Verification items for the finished model (mm, model axes). Face numbers are marked on the shaded views. A direction names the side the tool comes from. Round coordinates to 2 decimals unless told otherwise and drop trailing zeros. Write each loop counter-clockwise with the first axis right and the second up, starting at its lowest first coordinate (ties: lowest second). Pieces come first, ordered by that corner, then holes. Notation, with made-up numbers: (-11, 83) - (40, 83) arc R21 cw to (40, 88) - close; hole circle Ø1 at (57, 29.25). An arc over 180 degrees is marked (long way). Answer as a JSON object with one key per item and string values.
```python
from build123d import *

# Parameters (mm, degrees)
BOSS_EXTRUDE1_DEPTH = 5
SKETCH6_R           = 7
SKETCH6_R_2         = 2.25
CUT_EXTRUDE1_DEPTH  = 91.496055715
BOSS_EXTRUDE2_DEPTH = 10
SKETCH11_R          = 2.59
CUT_EXTRUDE3_DEPTH  = 3
SKETCH16_R          = 1.5
CUT_EXTRUDE6_DEPTH  = 119.415100811
SKETCH24_W          = 10
SKETCH24_H          = 50
BOSS_EXTRUDE8_DEPTH = 40
SKETCH25_R          = 7
CUT_EXTRUDE10_DEPTH = 132.23313644
SKETCH26_R          = 1.55
CUT_EXTRUDE11_DEPTH = 132.23313644


with BuildPart() as part:
    # Sketch3 → Boss-Extrude1 (new, symmetric)
    with BuildSketch(Plane.XY):
        with BuildLine():
            Line((0, 20), (87.69, 20))
            Line((87.69, 20), (87.69, -20))
            Line((87.69, -20), (0, -20))
            ThreePointArc((0, -20), (-20, 0), (0, 20))
        make_face()
    extrude(amount=BOSS_EXTRUDE1_DEPTH, both=True)

    # Sketch6 → Cut-Extrude1 (cut, through all)
    with BuildSketch(Plane.XY.offset(5)):
        with Locations((20, 0)):
            Circle(SKETCH6_R)
        with Locations((20, 11)):
            Circle(SKETCH6_R_2)
        with Locations((31, 0)):
            Circle(SKETCH6_R_2)
        with Locations((20, -11)):
            Circle(SKETCH6_R_2)
        with Locations((9, 0)):
            Circle(SKETCH6_R_2)
    extrude(amount=-CUT_EXTRUDE1_DEPTH, mode=Mode.SUBTRACT)

    # Sketch9 → Boss-Extrude2 (add)
    with BuildSketch(Plane(origin=(87.69, 0, 0), x_dir=(0, 0, -1), z_dir=(1, 0, 0))):
        Polygon((5, 20), (45, 20), (45, -20), (5, -20), (-5, -20), (-5, 20), align=None)
    extrude(amount=-BOSS_EXTRUDE2_DEPTH)

    # Sketch11 → Cut-Extrude3 (cut)
    with BuildSketch(Plane.XY.offset(5)):
        with Locations((-12, -1.375)):
            Circle(SKETCH11_R)
    extrude(amount=-CUT_EXTRUDE3_DEPTH, mode=Mode.SUBTRACT)

    # Sketch16 → Cut-Extrude6 (cut, through all)
    with BuildSketch(Plane(origin=(87.69, 0, 0), x_dir=(0, 0, -1), z_dir=(1, 0, 0))):
        with Locations((20, 16)):
            Circle(SKETCH16_R)
        with Locations((20, -2)):
            Circle(SKETCH16_R)
    extrude(amount=-CUT_EXTRUDE6_DEPTH, mode=Mode.SUBTRACT)

    # Sketch24 → Boss-Extrude8 (add)
    with BuildSketch(Plane(origin=(0, -20, 0), x_dir=(-1, 0, 0), z_dir=(0, -1, 0))):
        with Locations((-82.69, 20)):
            Rectangle(SKETCH24_W, SKETCH24_H)
    extrude(amount=BOSS_EXTRUDE8_DEPTH)

    # Sketch25 → Cut-Extrude10 (cut, through all)
    with BuildSketch(Plane(origin=(87.69, 0, 0), x_dir=(0, 0, -1), z_dir=(1, 0, 0))):
        with Locations((20, -40)):
            Circle(SKETCH25_R)
    extrude(amount=-CUT_EXTRUDE10_DEPTH, mode=Mode.SUBTRACT)

    # Sketch26 → Cut-Extrude11 (cut, through all)
    with BuildSketch(Plane(origin=(87.69, 0, 0), x_dir=(0, 0, -1), z_dir=(1, 0, 0))):
        with Locations((2.78, -24.223522787)):
            Circle(SKETCH26_R)
        with Locations((37.22, -24.223522787)):
            Circle(SKETCH26_R)
        with Locations((37.22, -55.223522787)):
            Circle(SKETCH26_R)
        with Locations((2.78, -55.223522787)):
            Circle(SKETCH26_R)
    extrude(amount=-CUT_EXTRUDE11_DEPTH, mode=Mode.SUBTRACT)


solid = part.part
```
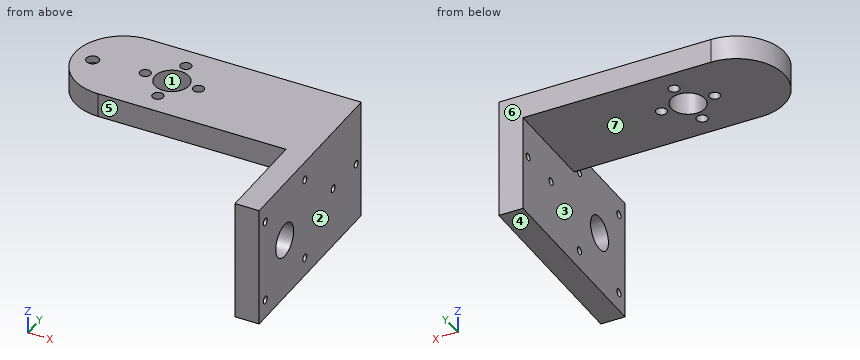
1. Cross-section at D-D (y = 16). Record the boundary of the cut face in (x, z), plus the area to 3 significant figures.
Completed:
{"outline": "(-12, -5) - (77.69, -5) - (77.69, -18.5) - (87.69, -18.5) - (87.69, 5) - (-12, 5) - close; (77.69, -45) - (87.69, -45) - (87.69, -21.5) - (77.69, -21.5) - close", "area": "1,370 mm^2"}
2. Material ranges on probe 1 along Y at (x, z) = (20, 1.5); probe 2 along Y at (x, z) = (80.5, -2.78); probe 3 along Z at (x, y) = (77, -17), recorded low to high. Write a range as from..to.
Completed:
{"probe 1": "y = -20..-13.25, -8.75..-7, 7..8.75, 13.25..20", "probe 2": "y = -60..-56.77, -53.67..-25.77, -22.67..20", "probe 3": "z = -5..5"}
3. Cross-section at B-B (x = 31). Record the boundary of the cut face in (y, z).
Completed:
{"outline": "(-20, -5) - (-2.25, -5) - (-2.25, 5) - (-20, 5) - close; (2.25, -5) - (20, -5) - (20, 5) - (2.25, 5) - close"}
4. Cross-section at A-A (z = -2.78). Record the boundary of the cut face in (x, y).
Completed:
{"outline": "(0, -20) - (77.69, -20) - (77.69, -22.67) - (87.69, -22.67) - (87.69, 20) - (0, 20) arc R20 ccw to start; (77.69, -60) - (87.69, -60) - (87.69, -56.77) - (77.69, -56.77) - close; (77.69, -53.67) - (87.69, -53.67) - (87.69, -25.77) - (77.69, -25.77) - close; hole circle Ø4.5 at (9, 0); hole circle Ø14 at (20, 0); hole circle Ø4.5 at (20, -11); hole circle Ø4.5 at (20, 11); hole circle Ø4.5 at (31, 0)"}
5. Cross-section at C-C (z = -20). Record the boundary of the cut face in (x, y), plus the area to 3 significant figures.
Completed:
{"outline": "(77.69, -60) - (87.69, -60) - (87.69, -47) - (77.69, -47) - close; (77.69, -33) - (87.69, -33) - (87.69, -3.5) - (77.69, -3.5) - close; (77.69, -0.5) - (87.69, -0.5) - (87.69, 14.5) - (77.69, 14.5) - close; (77.69, 17.5) - (87.69, 17.5) - (87.69, 20) - (77.69, 20) - close", "area": "600 mm^2"}
6. Access from +Z, -Z, +X, -X, +Y, -Y to the whole of each face (thin tool, end or side, straight path). Record for the marked faces 5, 6 and 7.
Completed:
{"face 5": "+Z, -Z, -X, -Y", "face 6": "+Z, -Z, +X, -X, +Y", "face 7": "-Z, -X, +Y, -Y"}
7. Mould release check, pull along X, two halves, no side actions. Record for the marked faces 1, 2, 3 and 4: released by +X, released by -X, zero draft, split by the parting line, or undercut.
Completed:
{"face 1": "undercut", "face 2": "released by +X", "face 3": "released by -X", "face 4": "zero draft"}
8. Go/stop test with flat-tipped pins: pin 1 (12 mm diameter, centred on x = 5, y = -5.5, fed in from -Z); pin 2 (8 mm diameter, centred on x = 55.5, z = -2, fed in from -Y); pin 3 (6 mm diameter, centred on y = -2.5, z = -14, fed in from -X). Record where each tip stops, or that it passes through.
Completed:
{"pin 1": "stops at z = -5", "pin 2": "stops at y = -20", "pin 3": "stops at x = 77.69"}
